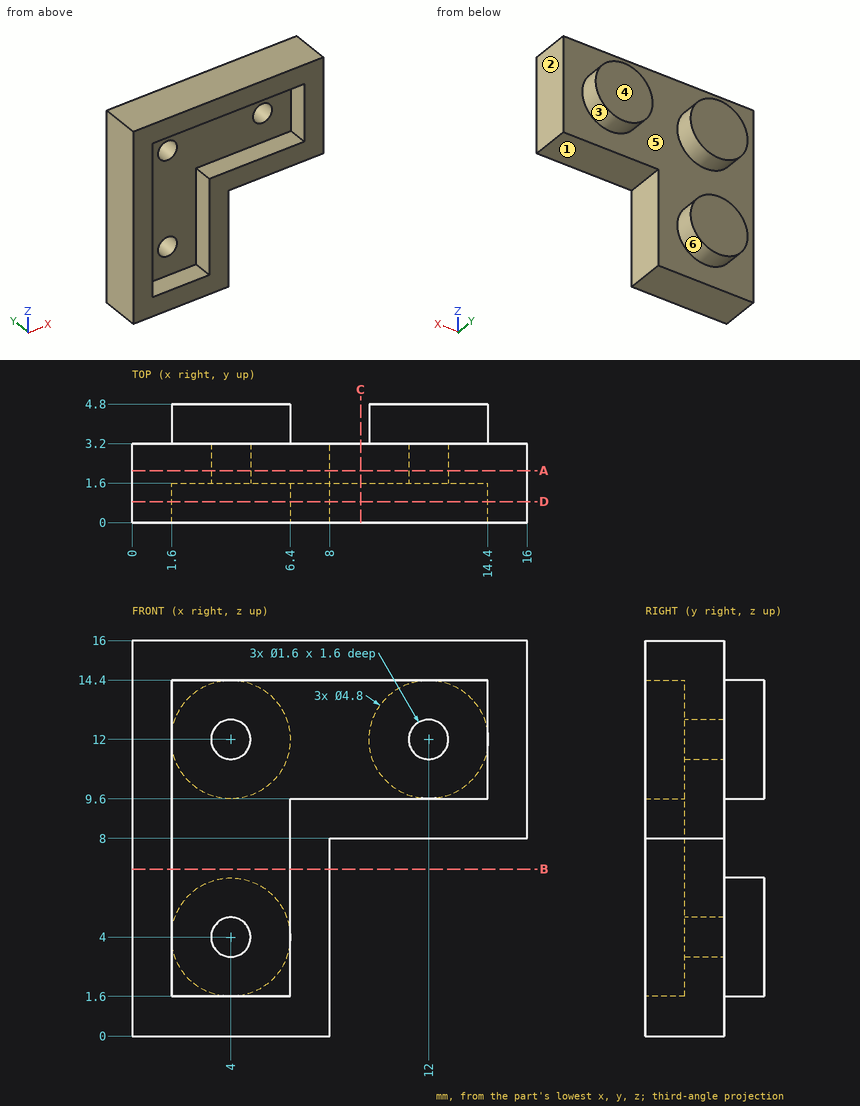
Geometry: see drawing. Coordinates: mm, zero at the bounding-box minimum. A direction names the side the tool comes from. Coordinates: 2 decimals unless noted, no trailing zeros. Write each loop counter-clockwise with the first axis right and the second up, starting at its lowest first coordinate (ties: lowest second). Pieces come first, ordered by that corner, then holes. Notation, with made-up numbers: (75, 44) - (87, 44) arc R17 cw to (87, 50) - close; hole circle Ø3 at (69.5, -16). An arc over 180 degrees is marked (long way). Put each result on its own line as item: value. Start each with the question number.
1) Reachability of the marked faces 1, 2 and 3 from +Z, -Z, +X, -X, +Y, -Y: full face, straight path, thin tool, end or side. Return the list, or none.
2) Cut plane C-C (x = 9.25). Return the cut outline in (y, z), plus the area to 3 significant figures.
3) Mould query, pull axis X, two halves, no side actions, for the marked faces 4, 5 and 6. Classes: pulls with the +X half, pulls with the -X half, needs draft (parallel to the pull), parting line crosses it, or undercut.
4) Ray query, L1, parallel to X at y = 2.45, z = 12; L2, parallel to Z at x = 8.75, y = 0.5; L3, parallel to X at y = 1.3, z = 11. Return the intervals inside material, ascending.
5) Cut plane B-B (z = 6.75). Return the cut outline in (x, y).
6) Contact query for flat-ended pins moving along their axis: pin 1 (6.5 mm diameter, centred on x = 7.5, z = 9.5, fed in from -Y); pin 2 (1.3 mm diameter, centred on x = 12, z = 12, fed in from -Y); pin 3 (0.8 mm diameter, centred on x = 4, z = 3.5, fed in from -Y); pin 4 (1 mm diameter, centred on y = 2.5, z = 3, fed in from +X). Output: stop coordinate, or through.
7) Cut plane D-D (y = 0.85). Return the cut outline in (x, z), plus the area to 3 significant figures.
8) Cut plane A-A (y = 2.1). Return the cut outline in (x, z).
Resolved:
1. face 1: -Z, +X, +Y, -Y
1. face 2: +Z, -Z, +X, +Y, -Y
1. face 3: +Y
2. outline: (0, 8) - (3.2, 8) - (3.2, 16) - (0, 16) - (0, 14.4) - (1.6, 14.4) - (1.6, 9.6) - (0, 9.6) - close
2. area: 17.9 mm2
3. face 4: needs draft
3. face 5: undercut
3. face 6: parting line crosses it
4. L1: x = 0 to 3.2, 4.8 to 11.2, 12.8 to 16
4. L2: z = 8 to 9.6, 14.4 to 16
4. L3: x = 0 to 1.6, 14.4 to 16
5. outline: (0, 0) - (1.6, 0) - (1.6, 1.6) - (6.4, 1.6) - (6.4, 0) - (8, 0) - (8, 3.2) - (0, 3.2) - close
6. pin 1: stops at y = 0
6. pin 2: stops at y = 3.2
6. pin 3: stops at y = 1.6
6. pin 4: stops at x = 8
7. outline: (0, 0) - (8, 0) - (8, 8) - (16, 8) - (16, 16) - (0, 16) - close; hole (1.6, 1.6) - (6.4, 1.6) - (6.4, 9.6) - (14.4, 9.6) - (14.4, 14.4) - (1.6, 14.4) - close
7. area: 92.2 mm2
8. outline: (0, 0) - (8, 0) - (8, 8) - (16, 8) - (16, 16) - (0, 16) - close; hole circle Ø1.6 at (4, 4); hole circle Ø1.6 at (4, 12); hole circle Ø1.6 at (12, 12)
